Verification items for this drawing (mm, ordinates from the low corner). A direction names the side the tool comes from. Coordinates: 2 decimals unless noted, no trailing zeros. Write each loop counter-clockwise with the first axis right and the second up, starting at its lowest first coordinate (ties: lowest second). Pieces come first, ordered by that corner, then holes. Notation, with made-up numbers: (-36, 23.5) -> (3, 23.5) arc R15 cw to (3, 42.5) -> close; hole circle Ø2 at (79.5, 13.5). An arc over 180 degrees is marked (long way). Answer as CSV lines item,"result".
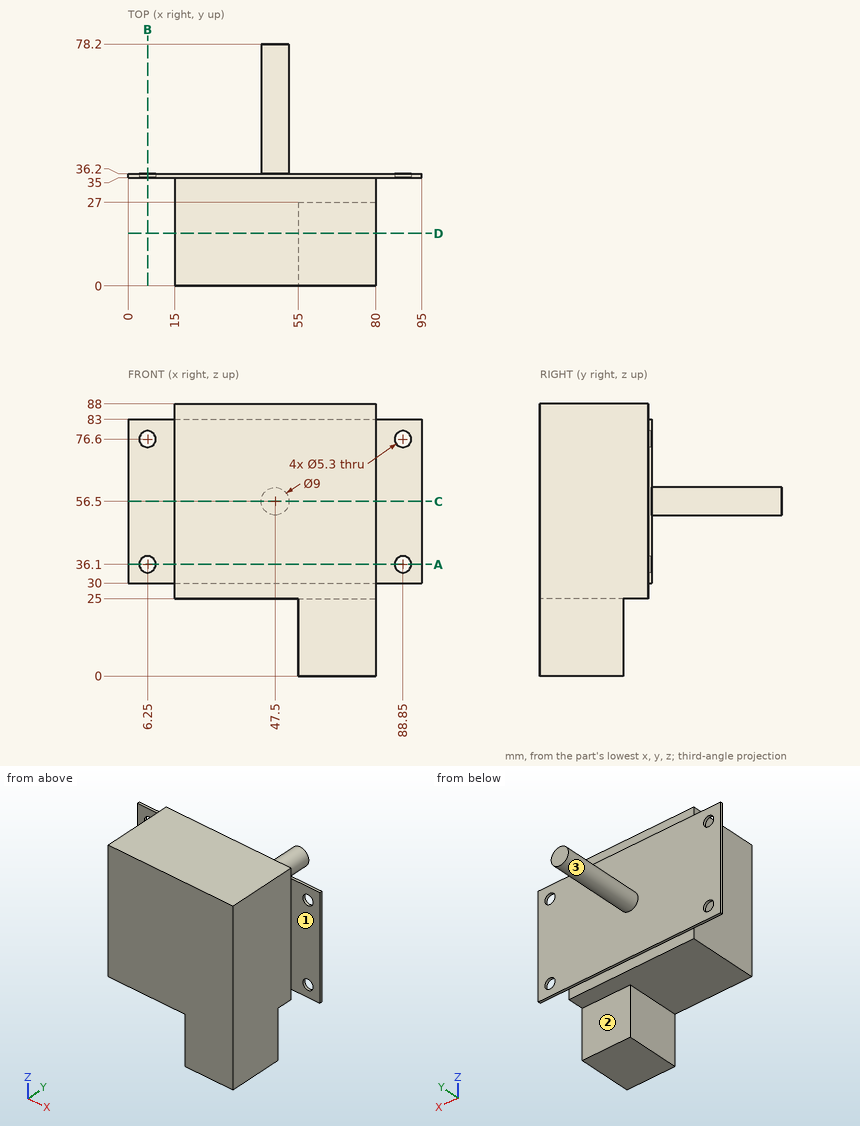
Item 1: Cross-section at D-D, the plane y = 17. Record the cut outline in (x, z), plus the area to 3 significant figures.
Responses:
outline,"(15, 25) -> (55, 25) -> (55, 0) -> (80, 0) -> (80, 88) -> (15, 88) -> close"
area,"4,720 mm2"
Item 2: Set-up check for the marked faces 1, 2 and 3: record each of +Z, -Z, +X, -X, +Y, -Y from which the full face is reachable in a straight line by a thin tool's end or side.
Responses:
face 1,"+Z, -Z, +X, -Y"
face 2,"-Z, +X, -X, +Y"
face 3,"+Y"
Item 3: Cross-section at C-C, the plane z = 56.5. Record the cut outline in (x, y).
Responses:
outline,"(0, 35) -> (15, 35) -> (15, 0) -> (80, 0) -> (80, 35) -> (95, 35) -> (95, 36.2) -> (52, 36.2) -> (52, 78.2) -> (43, 78.2) -> (43, 36.2) -> (0, 36.2) -> close"
Item 4: Cross-section at B-B, the plane x = 6.25. Record the cut outline in (y, z).
Responses:
outline,"(35, 30) -> (36.2, 30) -> (36.2, 33.45) -> (35, 33.45) -> close; (35, 38.75) -> (36.2, 38.75) -> (36.2, 73.95) -> (35, 73.95) -> close; (35, 79.25) -> (36.2, 79.25) -> (36.2, 83) -> (35, 83) -> close"
Item 5: Cross-section at A-A, the plane z = 36.1. Record the cut outline in (x, y), plus the area to 3 significant figures.
Responses:
outline,"(0, 35) -> (3.6, 35) -> (3.6, 36.2) -> (0, 36.2) -> close; (8.9, 35) -> (15, 35) -> (15, 0) -> (80, 0) -> (80, 35) -> (86.2, 35) -> (86.2, 36.2) -> (8.9, 36.2) -> close; (91.5, 35) -> (95, 35) -> (95, 36.2) -> (91.5, 36.2) -> close"
area,"2,380 mm2"
Item 6: Depth check by flat-ended pin: pin 1 Ø5 at (y, z) = (20.5, 72.5) entering from +X; pin 2 Ø1.5 at (x, z) = (10.5, 73.5) entering from -Y; pin 3 Ø1.3 at (x, y) = (53, 35.5) entering from +Z; pin 4 Ø1 at (x, z) = (69, 28) entering from +Y. Enter the tip coordinate at first touch or a pass-through.
Responses:
pin 1,"stops at x = 80"
pin 2,"stops at y = 35"
pin 3,"stops at z = 88"
pin 4,"stops at y = 35"
Item 7: Thickness scan on probe 1 along Z at (x, y) = (88.85, 35.75); probe 2 along Z at (x, y) = (44, 29); probe 3 along Z at (x, y) = (10.5, 36). Record the ranges inside material, lowest first.
Responses:
probe 1,"z = 30 to 33.45, 38.75 to 73.95, 79.25 to 83"
probe 2,"z = 25 to 88"
probe 3,"z = 30 to 83"
